Check sheet for the modelled part. Datum: model origin and axes. Units: mm. A direction names the side the tool comes from. Give positions to 0.01 mm unless a question says otherwise; leave off trailing zeros. Order: outer loops, then holes, each group sorted by start corner. A loop starts at its lowest first (then second) coordinate and runs counter-clockwise, first axis right, second up. Notation, with made-up numbers: (26, 66.25) - (70, 66.25) arc R30 ccw to (70, 100.25) - close; hole circle Ø9 at (11.25, 58.5). An arc over 180 degrees is marked (long way). Answer in a Markdown table with one row per item.
from build123d import *

# Parameters (mm, degrees)
F1_DEPTH  = 177.8
F2_DEPTH  = 304.8
F3_DEPTH  = 304.8
F4_DEPTH  = 304.8
F5_DEPTH  = 304.8
F6_DEPTH  = 304.8
F7_DEPTH  = 19.05
F9_DEPTH  = 304.8
F10_W     = 495.3
F10_H     = 120.65
F11_DEPTH = 19.05


with BuildPart() as f1:
    # F0 (on Top) → F1 (new body)
    with BuildSketch(Plane.XY):
        Polygon((-112.158418, 206.345618), (-101.6, 187.295618), (101.6, 187.295618), (112.184372, 206.304091), (112.158418, 206.345618), align=None)
    extrude(amount=F1_DEPTH)

    # F0 (on Top) → F2 (join)
    with BuildSketch(Plane.XY):
        Polygon((-247.65, -10.440914), (-228.6, -15.904382), (-101.6, 187.295618), (-112.158418, 206.345618), align=None)
    extrude(amount=F2_DEPTH)

    # F0 (on Top) → F3 (join)
    with BuildSketch(Plane.XY):
        Polygon((101.6, 187.295618), (228.6, -15.904382), (247.65, -10.440914), (112.184372, 206.304091), align=None)
    extrude(amount=F3_DEPTH)

    # F0 (on Top) → F4 (join)
    with BuildSketch(Plane.XY):
        Polygon((-247.65, -136.554382), (-228.6, -117.504382), (-228.6, -15.904382), (-247.65, -10.440914), align=None)
    extrude(amount=F4_DEPTH)

    # F0 (on Top) → F5 (join)
    with BuildSketch(Plane.XY):
        Polygon((228.6, -15.904382), (228.6, -117.504382), (247.65, -136.554382), (247.65, -10.440914), align=None)
    extrude(amount=F5_DEPTH)

    # F0 (on Top) → F6 (join)
    with BuildSketch(Plane.XY):
        Polygon((228.6, -117.504382), (-228.6, -117.504382), (-247.65, -136.554382), (247.65, -136.554382), align=None)
    extrude(amount=F6_DEPTH)

    # F0 (on Top) → F7 (join)
    with BuildSketch(Plane.XY):
        Polygon((-228.6, -15.904382), (-228.6, -117.504382), (228.6, -117.504382), (228.6, -15.904382), (101.6, 187.295618), (-101.6, 187.295618), align=None)
    extrude(amount=F7_DEPTH)

    # F8 (on Right) → F9 (cut, symmetric)
    with BuildSketch(Plane.YZ):
        Polygon((-12.7, 311.536975), (-12.7, 304.8), (208.28, 152.4), (208.28, 311.536975), align=None)
    extrude(amount=F9_DEPTH, both=True, mode=Mode.SUBTRACT)

    # F10 (on face) → F11 (join)
    with BuildSketch(Plane.XY.offset(304.8)):
        with Locations((0, -76.229382)):
            Rectangle(F10_W, F10_H)
    extrude(amount=-F11_DEPTH)


solid = f1.part
(1) Cross-section at A-A, the plane z = 124.5. Record the cut outline in (x, y), then the cut area to 3 significant figures.
Geometry says:
| item | result |
|---|---|
| outline | (-247.65, -136.55) - (247.65, -136.55) - (247.65, -10.44) - (112.18, 206.3) - (112.16, 206.35) - (-112.16, 206.35) - (-247.65, -10.44) - close; hole (-228.6, -117.5) - (228.6, -117.5) - (228.6, -15.9) - (101.6, 187.3) - (-101.6, 187.3) - (-228.6, -15.9) - close |
| area | 26,900 mm² |
(2) Gauge pin test, flat ends, axial feed: P1, Ø1.5, axis at y = 112.5, z = 130, coming from the +X side; P2, Ø6, axis at y = 165.5, z = 139.5, coming from the +X side; P3, Ø1.5, axis at x = 121, z = 78.5, coming from the +Y side; P4, Ø6, axis at x = 38, y = 17.5, coming from the -Z side. Record the tip position at first contact, or that the pin passes through.
Geometry says:
| item | result |
|---|---|
| P1 | x = 171.28 |
| P2 | x = 139.56 |
| P3 | y = 193.4 |
| P4 | z = 0 |
(3) Cross-section at C-C, the plane x = 140. Record the cut outline in (y, z).
Geometry says:
| item | result |
|---|---|
| outline | (-136.55, 0) - (161.8, 0) - (161.8, 184.46) - (125.86, 209.24) - (125.86, 19.05) - (-117.5, 19.05) - (-117.5, 285.75) - (-15.9, 285.75) - (-15.9, 304.8) - (-136.55, 304.8) - close |
(4) Cross-section at B-B, the plane y = 86. Record the cut outline in (x, z), then the cut area to 3 significant figures.
Geometry says:
| item | result |
|---|---|
| outline | (-187.37, 0) - (187.37, 0) - (187.37, 236.73) - (164.91, 236.73) - (164.91, 19.05) - (-164.91, 19.05) - (-164.91, 236.73) - (-187.37, 236.73) - close |
| area | 16,900 mm² |
(5) Mould release check, pull along Y, two halves, no side actions. Record for faces 4 (the flat face through (3, -117.504, 151)), 5 (the flat face through (-178.956, 99.47, 115.805)), 6 (the flat face through (-3, 37, 0)): pulls with the +Y half, pulls with the -Y half, needs draft (parallel to the pull), parting line crosses it, or undercut.
Geometry says:
| item | result |
|---|---|
| face 4 | undercut |
| face 5 | pulls with the +Y half |
| face 6 | needs draft |
(6) Access from +Z, -Z, +X, -X, +Y, -Y to the whole of each face (thin tool, end or side, straight path). Record for faces 1 (the flat face through (228.6, -66, 151)), 2 (the flat face through (-1, 187.296, 92)), 3 (the flat face through (1.156, 193.665, 162.479)).
Geometry says:
| item | result |
|---|---|
| face 1 | none |
| face 2 | +Z |
| face 3 | +Z, +X, -X, +Y |
(7) Cross-section at D-D, the plane z = 229. Record the cut outline in (x, y), then the cut area to 3 significant figures.
Geometry says:
| item | result |
|---|---|
| outline | (-247.65, -136.55) - (247.65, -136.55) - (247.65, -10.44) - (180.37, 97.21) - (157.9, 97.21) - (228.6, -15.9) - (228.6, -117.5) - (-228.6, -117.5) - (-228.6, -15.9) - (-157.9, 97.21) - (-180.37, 97.21) - (-247.65, -10.44) - close |
| area | 18,400 mm² |
(8) Thickness scan on L1, parallel to X at y = -106, z = 204; L2, parallel to Z at x = 114.5, y = -24; L3, parallel to Y at x = -64, z = 29.5. Record the ranges inside material, lowest first.
Geometry says:
| item | result |
|---|---|
| L1 | -247.65 to -228.6, 228.6 to 247.65 |
| L2 | 0 to 19.05, 285.75 to 304.8 |
| L3 | -136.55 to -117.5, 187.3 to 206.35 |
